Could you check a few things on this model? Use its own coordinates, in mm. Coordinates: 2 decimals unless noted, no trailing zeros. Answer as a JSON object with one key per item and string values. Group by question number.
(1) Please list where these lines run through material, in increasing order: probe 1 along Y at (x, z) = (-14.25, -15); probe 2 along Y at (x, z) = (-35, -14.25); probe 3 along Y at (x, z) = (-44, -13.5).
(2) Will these pins go through, and if not, where does the flat tip stop? P1, Ø5.5, axis at y = 30, z = -15, coming from the +X side; P2, Ø6.5, axis at y = 135, z = -15, coming from the -X side; P3, Ø8.5, axis at y = 535, z = -15, coming from the -X side.
(3) We'd pull the mould along X, two halves only. Please class faces 1 (the flat face through (0, 345, -15)), 2 (the flat face through (-50, 345, -15)), 3 (the flat face through (-25, 700, -15)): pulls with the +X half, pulls with the -X half, needs draft (parallel to the pull), parting line crosses it, or undercut.
from build123d import *

# Parameters (mm, degrees)
SKETCH_1_W       = 50
SKETCH_1_H       = 700
EXTRUDE_1_DEPTH  = 30
M10X1_25_1_D     = 8.8
M10X1_25_1_DEPTH = 23.75
M10X1_25_1_TIP   = 2.643786724
M12X1_5_1_D      = 10.5
M12X1_5_1_DEPTH  = 28.5
M12X1_5_1_TIP    = 3.15451825


with BuildPart() as part:
    # 草图1 → 凸台-拉伸1 (new body)
    with BuildSketch(Plane.XY):
        with Locations((-25, 350)):
            Rectangle(SKETCH_1_W, SKETCH_1_H)
    extrude(amount=-EXTRUDE_1_DEPTH)

    # M10x1.25 螺纹孔1
    with Locations(Plane(origin=(0, 0, 0), x_dir=(0, 0, -1), z_dir=(1, 0, 0))):
        with Locations((15, 670), (15, 450), (15, 250), (15, 30)):
            Hole(M10X1_25_1_D / 2, depth=M10X1_25_1_DEPTH)
            with Locations((0, 0, -(M10X1_25_1_DEPTH + M10X1_25_1_TIP / 2))):  # 118° drill point
                Cone(0, M10X1_25_1_D / 2, M10X1_25_1_TIP, mode=Mode.SUBTRACT)

    # M12x1.5 螺纹孔1
    with Locations(Plane.ZY.offset(50)):
        with Locations((-15, 535), (-15, 135)):
            Hole(M12X1_5_1_D / 2, depth=M12X1_5_1_DEPTH)
            with Locations((0, 0, -(M12X1_5_1_DEPTH + M12X1_5_1_TIP / 2))):  # 118° drill point
                Cone(0, M12X1_5_1_D / 2, M12X1_5_1_TIP, mode=Mode.SUBTRACT)


solid = part.part
Result set:
{
 "1": {"probe 1": "y = 0 to 25.6, 34.4 to 245.6, 254.4 to 445.6, 454.4 to 665.6, 674.4 to 700", "probe 2": "y = 0 to 129.8, 140.2 to 529.8, 540.2 to 700", "probe 3": "y = 0 to 129.97, 140.03 to 529.97, 540.03 to 700"},
 "2": {"P1": "stops at x = -24.74", "P2": "stops at x = -20.3", "P3": "stops at x = -20.9"},
 "3": {"face 1": "pulls with the +X half", "face 2": "pulls with the -X half", "face 3": "needs draft"}
}
